Verification items for the finished model (mm, model axes). Face numbers are marked on the shaded views. Round coordinates to 2 decimals unless told otherwise and drop trailing zeros. Order: outer loops, then holes, each group sorted by start corner. A loop starts at its lowest first (then second) coordinate and runs counter-clockwise, first axis right, second up. Notation, with made-up numbers: (78.25, -38) -> (125.25, -38) arc R18 ccw to (125.25, -19) -> close; hole circle Ø2 at (-9, -29). An arc over 180 degrees is marked (long way). Put each result on its own line as item: value.
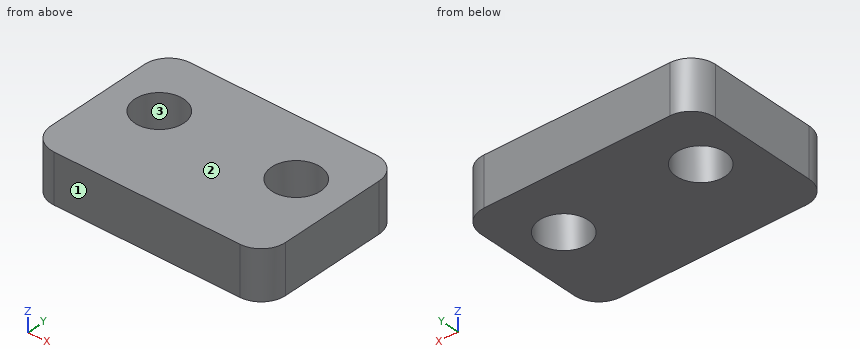
```python
from build123d import *

# Parameters (mm, degrees)
F0_W     = 96
F0_H     = 64
F1_DEPTH = 20
F2_R     = 10
F3_R     = 10
F4_DEPTH = 25
F5_DEPTH = 55.9


with BuildPart() as f1:
    # F0 (on Top) → F1 (new body)
    with BuildSketch(Plane.XY):
        Rectangle(F0_W, F0_H)
    extrude(amount=F1_DEPTH)

    # F2
    f2_edges = [f1.edges().sort_by_distance(p)[0] for p in [
        (48, -32, 10),
        (48, 32, 10),
        (-48, 32, 10),
        (-48, -32, 10),
    ]]
    fillet(f2_edges, radius=F2_R)

    # F3 (on face) → F4 (cut)
    with BuildSketch(Plane.XY.offset(20)):
        with Locations((28, 6)):
            Circle(F3_R)
    extrude(amount=-F4_DEPTH, mode=Mode.SUBTRACT)

    # F3 (on face) → F5 (cut)
    with BuildSketch(Plane.XY.offset(20)):
        with Locations((-28, 6)):
            Circle(F3_R)
    extrude(amount=-F5_DEPTH, mode=Mode.SUBTRACT)


solid = f1.part
```
Item 1: Sectioned sample at A-A, the plane y = 6. Record the boundary of the cut face in (x, z).
Geometry check:
outline: (-48, 0) -> (-38, 0) -> (-38, 20) -> (-48, 20) -> close; (-18, 0) -> (18, 0) -> (18, 20) -> (-18, 20) -> close; (38, 0) -> (48, 0) -> (48, 20) -> (38, 20) -> close
Item 2: Sectioned sample at D-D, the plane y = -28. Record the boundary of the cut face in (x, z), then the cut area to 3 significant figures.
Geometry check:
outline: (-46, 0) -> (46, 0) -> (46, 20) -> (-46, 20) -> close
area: 1,840 mm2
Item 3: Depth check by flat-ended pin: pin 1 Ø16 at (x, y) = (28, 6) entering from -Z. Enter the tip coordinate at first touch or a pass-through.
Geometry check:
pin 1: through
Item 4: Release check for a two-part mould opening along Y. For the marked faces 1, 2 and 3 record: pulls with the +Y half, pulls with the -Y half, needs draft (parallel to the pull), parting line crosses it, or undercut.
Geometry check:
face 1: pulls with the -Y half
face 2: needs draft
face 3: undercut
Item 5: Sectioned sample at B-B, the plane x = 27. Record the boundary of the cut face in (y, z).
Geometry check:
outline: (-32, 0) -> (-3.95, 0) -> (-3.95, 20) -> (-32, 20) -> close; (15.95, 0) -> (32, 0) -> (32, 20) -> (15.95, 20) -> close
Item 6: Sectioned sample at C-C, the plane z = 2.5. Record the boundary of the cut face in (x, y), then the cut area to 3 significant figures.
Geometry check:
outline: (-48, -22) arc R10 ccw to (-38, -32) -> (38, -32) arc R10 ccw to (48, -22) -> (48, 22) arc R10 ccw to (38, 32) -> (-38, 32) arc R10 ccw to (-48, 22) -> close; hole circle Ø20 at (-28, 6); hole circle Ø20 at (28, 6)
area: 5,430 mm2
Item 7: Material ranges on line 1 along Y through (x, z) = (-28, 10.75); line 2 along X through (y, z) = (9.5, 18); line 3 along X through (y, z) = (4, 3), recorded low to high.
Geometry check:
line 1: -32 to -4, 16 to 32
line 2: -48 to -37.37, -18.63 to 18.63, 37.37 to 48
line 3: -48 to -37.8, -18.2 to 18.2, 37.8 to 48
